Here's how the part is built. I have some questions about the finished solid (model axes, mm). A direction names the side the tool comes from. Round coordinates to 2 decimals unless told otherwise and drop trailing zeros. Write each loop counter-clockwise with the first axis right and the second up, starting at its lowest first coordinate (ties: lowest second). Pieces come first, ordered by that corner, then holes. Notation, with made-up numbers: (-14, 62) - (23, 62) arc R25 ccw to (23, 93) - close; hole circle Ø5 at (-18.5, 70.5). An arc over 180 degrees is marked (long way). Write item = value, one per line. Start each with the question number.
Item 1: If we section it at D-D (x = 36.5): Please give me the cut outline in (y, z).
Item 2: For P1, Ø3, axis at x = -36, y = -7.5, coming from the -Z side; P2, Ø9, axis at x = -34.5, z = -7, coming from the -Y side, each with a flat end and sliding along its axis, tell me the tip position at first contact or that it passes through.
Item 3: If we section it at B-B (x = -38): Please give me the cut outline in (y, z).
Item 4: Thinking about a two-plate mould opening in X: for faces 1 (the face through (48.31, -7.4, -0.96)), 2 (the face through (46, -15, 0)), 3 (the face through (75, 5, 0)), which applies, pulls with the +X half, pulls with the -X half, needs draft (parallel to the pull), parting line crosses it, or undercut?
Item 5: If we section it at C-C (z = 0): Please give me the cut outline in (x, y), and give its area (4 significant figures).
Item 6: If we section it at A-A (y = -9.5): Please give me the cut outline in (x, z), and give its area (3 significant figures).
Item 7: Which directions (+Z, -Z, +X, -X, +Y, -Y) give clear straight access to the entire face, cutting with the end or side of a thin tool? Please do faces 4 (the face through (22, -15, 0)), 5 (the face through (-35.69, -7.4, -0.96)).
Item 8: If I drill on line 1 along Y through (x, z) = (59, 7.5); line 2 along Z through (x, y) = (-0.5, -0.75); line 3 along Z through (x, y) = (-36.5, -6), over which ranges is the centre line in solid material (lowest first)? Write a range as [from, to].
```python
from build123d import *

# Parameters (mm, degrees)
F0_W     = 150
F0_H     = 30
F1_DEPTH = 10
F2_R     = 2.5
F3_DEPTH = 15


with BuildPart() as f1:
    # F0 (on Front) → F1 (new body)
    with BuildSketch(Plane.XZ):
        Rectangle(F0_W, F0_H)
    extrude(amount=-F1_DEPTH)

    # F2 (on face) → F3 (join)
    with BuildSketch(Plane.XZ):
        with Locations((-38, 0)):
            Circle(F2_R)
        with Locations((-20, 0)):
            Circle(F2_R)
        Circle(F2_R)
        with Locations((22, 0)):
            Circle(F2_R)
        with Locations((46, 0)):
            Circle(F2_R)
    extrude(amount=F3_DEPTH)


solid = f1.part
```
Reply:
q1.outline = (0, -15) - (10, -15) - (10, 15) - (0, 15) - close
q2.P1 = -2.45
q2.P2 = 0
q3.outline = (-15, -2.5) - (0, -2.5) - (0, -15) - (10, -15) - (10, 15) - (0, 15) - (0, 2.5) - (-15, 2.5) - close
q4.face_1 = undercut
q4.face_2 = needs draft
q4.face_3 = pulls with the +X half
q5.outline = (-75, 0) - (-40.5, 0) - (-40.5, -15) - (-35.5, -15) - (-35.5, 0) - (-22.5, 0) - (-22.5, -15) - (-17.5, -15) - (-17.5, 0) - (-2.5, 0) - (-2.5, -15) - (2.5, -15) - (2.5, 0) - (19.5, 0) - (19.5, -15) - (24.5, -15) - (24.5, 0) - (43.5, 0) - (43.5, -15) - (48.5, -15) - (48.5, 0) - (75, 0) - (75, 10) - (-75, 10) - close
q5.area = 1,875 mm2
q6.outline = circle Ø5 at (-38, 0); circle Ø5 at (-20, 0); circle Ø5 at (0, 0); circle Ø5 at (22, 0); circle Ø5 at (46, 0)
q6.area = 98.2 mm2
q7.face_4 = +Z, -Z, +X, -X, -Y
q7.face_5 = -Y
q8.line_1 = [0, 10]
q8.line_2 = [-2.45, 2.45]
q8.line_3 = [-2, 2]
